Design review of the part built by this model. Coordinates are the model's own, in mm. A direction names the side the tool comes from. Give positions to 0.01 mm unless a question says otherwise; leave off trailing zeros. Write each loop counter-clockwise with the first axis right and the second up, starting at its lowest first coordinate (ties: lowest second). Pieces come first, ordered by that corner, then holes. Notation, with made-up numbers: M -16.5,86 L 10.5,86 A18 cw 10.5,105 Z; hole C 47.5,81.25 d5. An arc over 180 degrees is marked long. One line per item, written item: value. Start each with the question number.
```python
from build123d import *

# Parameters (mm, degrees)
F2_DEPTH = 88.9
F3_W     = 26.7864570916
F3_H     = 88.9
F4_DEPTH = 88.9


# Not quite as in the source:
# - a variable given as a bare number and used for a length is read in inches; the dataset says mm whatever the document's units were


with BuildPart() as f2:
    # F1 (on Front) → F2 (new body)
    with BuildSketch(Plane.XZ):
        with BuildLine():
            Line((85.6085425377, 530.4986528046), (34.8085425377, 530.4986528046))
            Line((34.8085425377, 530.4986528046), (-15.9914574623, 530.4986528046))
            Line((-15.9914574623, 530.4986528046), (-17.8685326312, 441.5986528046))
            ThreePointArc((-17.8685326312, 441.5986528046), (-192.6665275597, -8.6975481194), (-269.9914574623, -485.5013471954))
            Line((-269.9914574623, -485.5013471954), (-130.0577898718, -485.5013471954))
            ThreePointArc((-130.0577898718, -485.5013471954), (-77.615001681, -123.7260262863), (34.8085425377, 224.1138442826))
            ThreePointArc((34.8085425377, 224.1138442826), (147.2320867564, -123.7260262863), (199.6748749472, -485.5013471954))
            Line((199.6748749472, -485.5013471954), (339.6085425377, -485.5013471954))
            ThreePointArc((339.6085425377, -485.5013471954), (262.2836126351, -8.6975481194), (87.4856177066, 441.5986528046))
            Line((87.4856177066, 441.5986528046), (85.6085425377, 530.4986528046))
        make_face()
    extrude(amount=F2_DEPTH)

    # F3 (on face) → F4 (cut)
    with BuildSketch(Plane.XY.offset(530.4986528046)):
        Polygon((-15.9914574623, -88.9), (6.2335425377, -88.9), (-15.9914574623, 0), align=None)
        Polygon((85.6085425377, 0), (63.3835425377, -88.9), (85.6085425377, -88.9), align=None)
        Polygon((122.7087825537, 0), (85.6085425377, 0), (85.6085425377, -88.9), (129.0911585093, -88.9), align=None)
        with Locations((-29.3846860081, -44.45)):
            Rectangle(F3_W, F3_H)
    extrude(amount=-F4_DEPTH, mode=Mode.SUBTRACT)


solid = f2.part
```
Q1. The part is to be moulded in two halves that separate along X. For faces 1 (the face through (269, -44, -485.501)), 2 (the face through (74.65, -43.83, 486.67)), 3 (the face through (146.067, -43.828, -118.736)), say which applies: pulls with the +X half, pulls with the -X half, needs draft (parallel to the pull), parting line crosses it, or undercut.
Q2. Take a section at A-A, the plane z = 151. Give the boundary of the cut face in (x, y).
Q3. Take a section at B-B, the plane y = -48.5. Give the boundary of the cut face in (x, z), then the cut area to 3 significant figures.
Q4. Take a section at D-D, the plane x = -160.5. Give the boundary of the cut face in (y, z).
Q5. Take a section at C-C, the plane z = -277.5. Give the boundary of the cut face in (x, y).
Q6. Machinability: for faces 4 (the face through (-9, -54, 441.599)), 5 (the face through (81, -54, 441.599)), 6 (the face through (264.052, -43.828, -15.238)), which of the approach directions +Z, -Z, +X, -X, +Y, -Y give a long, thin tool a straight path to every point of the face, cutting with its end or side? Answer none if there is none.
Q7. Wall thickness on line 1 (X direction, y = -63, z = -387.5); line 2 (X direction, y = -11.5, z = -149); line 3 (X direction, y = -71, z = 265): over which ranges is each line inside the solid? List them lowest first. Write a range as from..to.
Q8. For P1, Ø8, axis at y = -10.5, z = -73.5, coming from the -X side; P2, Ø12, axis at x = 152, y = -56, coming from the +Z side; P3, Ø12, axis at y = -76.5, z = -239, coming from the +X side, all flat-tipped, find the tip position at first contact; note any pin that passes through.
Results list:
1. face 1: needs draft
1. face 2: pulls with the +X half
1. face 3: undercut
2. outline: M -142.96,-88.9 L 5.71,-88.9 L 5.71,0 L -142.96,0 Z; M 63.91,-88.9 L 212.58,-88.9 L 212.58,0 L 63.91,0 Z
3. outline: M -269.99,-485.5 L -130.06,-485.5 A2170.11 cw 34.81,224.11 A2170.11 cw 199.67,-485.5 L 339.61,-485.5 A2309.81 ccw 87.49,441.6 L 73.48,441.6 L 73.48,530.5 L -3.87,530.5 L -3.87,441.6 L -17.87,441.6 A2309.81 ccw Z
3. area: 256,000 mm^2
4. outline: M -88.9,-485.5 L 0,-485.5 L 0,99.14 L -88.9,99.14 Z
5. outline: M -248.85,-88.9 L -107.54,-88.9 L -107.54,0 L -248.85,0 Z; M 177.15,-88.9 L 318.47,-88.9 L 318.47,0 L 177.15,0 Z
6. face 4: +Z, -X, -Y
6. face 5: +Z, +X, -Y
6. face 6: +Z, +X, +Y, -Y
7. line 1: x = -262.4..-121.98, 191.59..332.02
7. line 2: x = -226.15..-83.33, 152.95..295.77
7. line 3: x = -99.48..169.1
8. P1: stops at x = -210.25
8. P2: stops at z = 319.1
8. P3: stops at x = 313.43
